```python
from build123d import *

# Parameters (mm, degrees)
SKETCH1_R           = 20.6375
SKETCH1_R_2         = 14.2875
BOSS_EXTRUDE2_DEPTH = 12.7
SKETCH2_R           = 3.175
CUT_EXTRUDE1_DEPTH  = 12.7


with BuildPart() as part:
    # Sketch1 → Boss-Extrude2 (new body)
    with BuildSketch(Plane.XY):
        with BuildLine():
            Line((-6.517989108, 18.562745695), (0, 0))
            Line((0, 0), (50.8, 0))
            Line((50.8, 0), (50.8, 46.0375))
            Line((50.8, 46.0375), (12.954, 46.0375))
            ThreePointArc((12.954, 46.0375), (27.546916197, 39.992916197), (33.5915, 25.4))
            ThreePointArc((33.5915, 25.4), (16.421941106, 5.055964247), (-6.517989108, 18.562745695))
        make_face()
        with Locations((12.954, 25.4)):
            Circle(SKETCH1_R)
        with Locations((12.954, 25.4)):
            Circle(SKETCH1_R_2, mode=Mode.SUBTRACT)
    extrude(amount=BOSS_EXTRUDE2_DEPTH)

    # Sketch2 → Cut-Extrude1 (cut)
    with BuildSketch(Plane.XZ):
        with Locations((45.085, 6.35)):
            Circle(SKETCH2_R)
        with Locations((5.715, 6.35)):
            Circle(SKETCH2_R)
    extrude(amount=-CUT_EXTRUDE1_DEPTH, mode=Mode.SUBTRACT)


solid = part.part
```
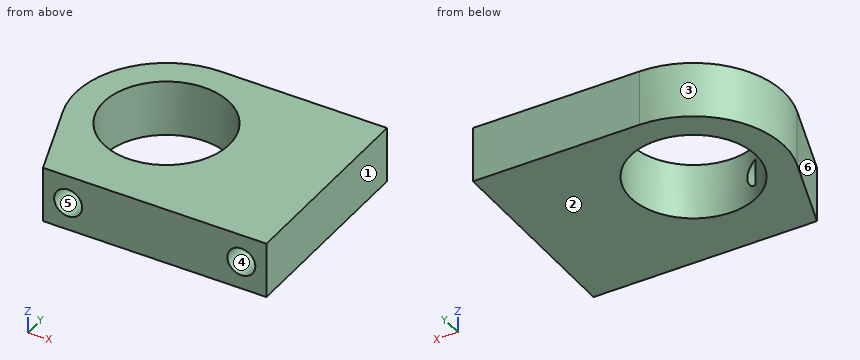
For this review, take the finished solid that the model builds, in its own axes (mm). Face numbers are marked on the shaded views. A direction names the side the tool comes from. Round coordinates to 2 decimals unless told otherwise and drop trailing zeros. Loops run counter-clockwise (first coordinate to the right, second up) from the corner with the lowest first, then second, coordinate; pieces in that order, holes last.
Q1. Add section A-A on y = 25.4. Write out the cut boundary in (x, z), plus the area to 3 significant figures.
Result sheet:
outline: (-7.68, 0) - (-1.33, 0) - (-1.33, 12.7) - (-7.68, 12.7) - close; (27.24, 0) - (50.8, 0) - (50.8, 12.7) - (27.24, 12.7) - close
area: 380 mm2
Q2. Machinability: for the marked faces 5 and 6, which of the approach directions +Z, -Z, +X, -X, +Y, -Y give a long, thin tool a straight path to every point of the face, cutting with its end or side? Answer none if there is none.
Result sheet:
face 5: -Y
face 6: +Z, -Z, -X, -Y
Q3. Add section B-B on x = 20.5. Write out the cut boundary in (y, z).
Result sheet:
outline: (0, 0) - (13.27, 0) - (13.27, 12.7) - (0, 12.7) - close; (37.53, 0) - (46.04, 0) - (46.04, 12.7) - (37.53, 12.7) - close
Q4. Add section D-D on z = 8.5. Write out the cut boundary in (x, y) (1 decimal).
Result sheet:
outline: (-6.5, 18.6) - (0, 0) - (3.4, 0) - (3.4, 12.7) - (6.4, 12.7) arc R14.3 cw (long way) to (8.1, 12) - (8.1, 0) - (42.7, 0) - (42.7, 12.7) - (47.4, 12.7) - (47.4, 0) - (50.8, 0) - (50.8, 46) - (13, 46) arc R20.6 ccw to start
Q5. To check wall thickness, follow line 1 along X through (y, z) = (26, 6); line 2 along Z through (x, y) = (44.5, 4); line 3 along Y through (x, z) = (17, 2.25). State the ranges of each line that lie inside material, in increasing order.
Result sheet:
line 1: x = -7.67 to -1.32, 27.23 to 50.8
line 2: z = 0 to 3.23, 9.47 to 12.7
line 3: y = 0 to 11.7, 39.1 to 46.04
Q6. Add section C-C on y = 10. Write out the cut boundary in (x, z) (3 decimals), plus the area to 3 significant figures.
Result sheet:
outline: (-3.511, 0) - (50.8, 0) - (50.8, 12.7) - (-3.511, 12.7) - close; hole circle Ø6.35 at (5.715, 6.35); hole circle Ø6.35 at (45.085, 6.35)
area: 626 mm2
Q7. Mouldability with a two-part tool opening along X and no side actions: class the marked faces 1, 2, 3 and 4 as +X half, -X half, draft (parallel to the pull), parting line (faces both ways), or undercut.
Result sheet:
face 1: +X half
face 2: draft
face 3: -X half
face 4: undercut
Q8. Insertion check: pin 1 Ø1.5 at (x, y) = (42.5, 18) entering from -Z; pin 2 Ø5.5 at (x, z) = (5.715, 6.35) entering from -Y; pin 3 Ø4 at (x, y) = (24.5, 22) entering from +Z. Each pin has a flat end and moves straight along its axis. Give the tip position at first contact, or say it passes through.
Result sheet:
pin 1: stops at z = 0
pin 2: stops at y = 12.7
pin 3: passes through
